Verification items for this drawing (mm, ordinates from the low corner). A direction names the side the tool comes from. Round coordinates to 2 decimals unless told otherwise and drop trailing zeros. Order: outer loops, then holes, each group sorted by start corner. A loop starts at its lowest first (then second) coordinate and runs counter-clockwise, first axis right, second up.
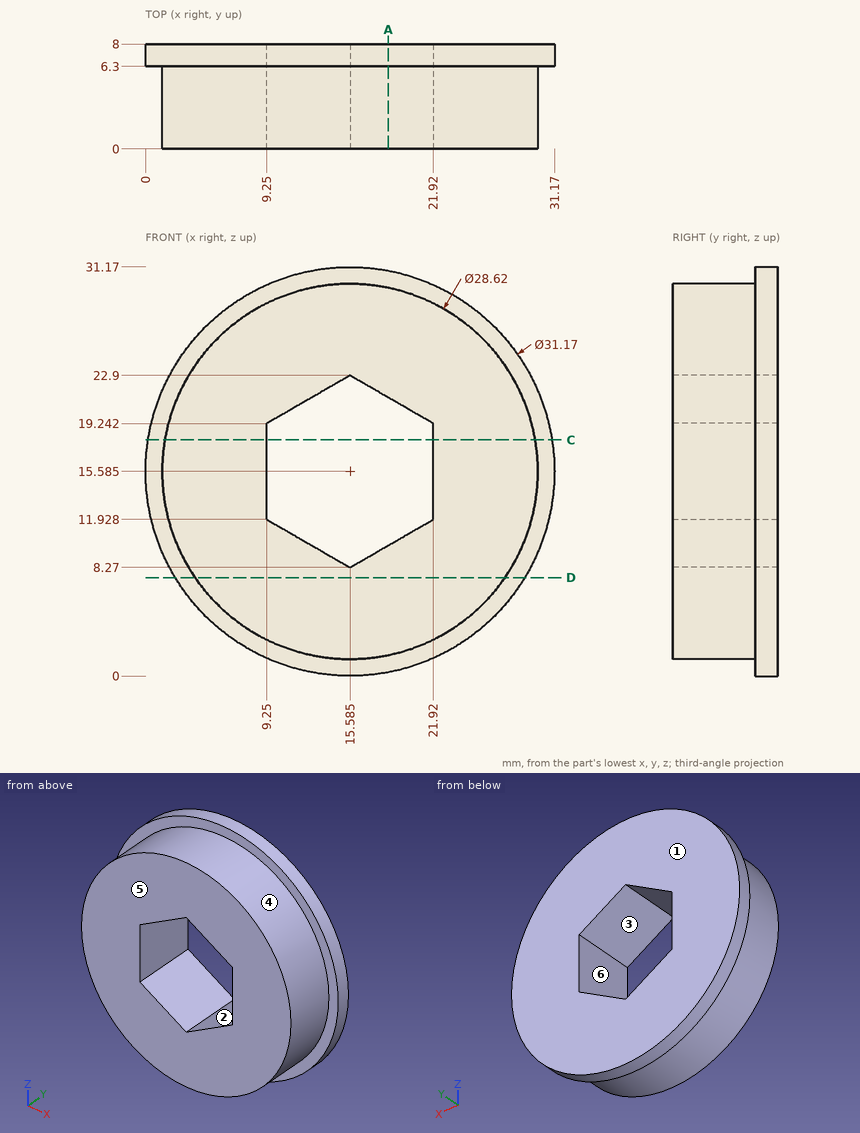
Item 1: Access from +Z, -Z, +X, -X, +Y, -Y to the whole of each face (thin tool, end or side, straight path). Record for the marked faces 1 and 2.
Answer:
face 1: +Z, -Z, +X, -X, +Y
face 2: +Y, -Y
Item 2: Sectioned sample at C-C (z = 18). Record the cut outline in (x, y).
Answer:
outline: (0.19, 6.3) - (1.48, 6.3) - (1.48, 0) - (9.25, 0) - (9.25, 8) - (0.19, 8) - close; (21.92, 0) - (29.69, 0) - (29.69, 6.3) - (30.98, 6.3) - (30.98, 8) - (21.92, 8) - close
Item 3: Release check for a two-part mould opening along X. For the marked faces 3, 4, 5 and 6 record: released by +X, released by -X, zero draft, split by the parting line, or undercut.
Answer:
face 3: undercut
face 4: split by the parting line
face 5: zero draft
face 6: undercut
Item 4: Go/stop test with flat-tipped pins: P1, Ø2, axis at y = 5, z = 16.5, coming from the -X side (1 decimal); P2, Ø2, axis at y = 5, z = 15, coming from the +X side (1 decimal); P3, Ø2, axis at y = 1, z = 23, coming from the -X side. Record where each tip stops, or that it passes through.
Answer:
P1: stops at x = 1.3
P2: stops at x = 29.9
P3: stops at x = 2.79
Item 5: Scan lines: line 1 along X through (y, z) = (1.75, 16); line 2 along Z through (x, y) = (19.5, 6.5); line 3 along Z through (x, y) = (14, 2.25) (1 decimal). Record each from-to range of solid material in increasing order.
Answer:
line 1: x = 1.28 to 9.25, 21.92 to 29.89
line 2: z = 0.5 to 10.53, 20.64 to 30.67
line 3: z = 1.4 to 9.2, 22 to 29.8
Item 6: Sectioned sample at D-D (z = 7.5). Record the cut outline in (x, y).
Answer:
outline: (2.26, 6.3) - (3.78, 6.3) - (3.78, 0) - (27.39, 0) - (27.39, 6.3) - (28.91, 6.3) - (28.91, 8) - (2.26, 8) - close
Item 7: Sectioned sample at A-A (x = 18.5). Record the cut outline in (y, z) (1 decimal).
Answer:
outline: (0, 1.6) - (6.3, 1.6) - (6.3, 0.3) - (8, 0.3) - (8, 10) - (0, 10) - close; (0, 21.2) - (8, 21.2) - (8, 30.9) - (6.3, 30.9) - (6.3, 29.6) - (0, 29.6) - close
